from build123d import *

# Parameters (mm, degrees)
SKETCH1_W           = 20
SKETCH1_H           = 20
BOSS_EXTRUDE1_DEPTH = 17
CUT_EXTRUDE1_DEPTH  = 17
SKETCH3_W           = 17
SKETCH3_H           = 13
CUT_EXTRUDE2_DEPTH  = 17
CUT_EXTRUDE3_REACH  = 35
SKETCH4_R           = 3.1
CUT_EXTRUDE4_REACH  = 35
SKETCH5_R           = 3.1


with BuildPart() as part:
    # Sketch1 → Boss-Extrude1 (new body)
    with BuildSketch(Plane(origin=(0, 0, 0), x_dir=(1, 0, 0), z_dir=(0, 1, 0))):
        with Locations((10, 10)):
            Rectangle(SKETCH1_W, SKETCH1_H)
    extrude(amount=BOSS_EXTRUDE1_DEPTH)

    # Sketch2 → Cut-Extrude1 (cut)
    with BuildSketch(Plane(origin=(0, 17, 0), x_dir=(1, 0, 0), z_dir=(0, 1, 0))):
        Polygon((3, 20), (20, 3), (20, 20), align=None)
    extrude(amount=-CUT_EXTRUDE1_DEPTH, mode=Mode.SUBTRACT)

    # Sketch3 → Cut-Extrude2 (cut)
    with BuildSketch(Plane(origin=(0, 0, -20), x_dir=(-1, 0, 0), z_dir=(0, 0, -1))):
        with Locations((-11.5, 8.5)):
            Rectangle(SKETCH3_W, SKETCH3_H)
    extrude(amount=-CUT_EXTRUDE2_DEPTH, mode=Mode.SUBTRACT)

    # Sketch4 → Cut-Extrude3 (cut, up to next)
    with BuildSketch(Plane.ZY, mode=Mode.PRIVATE) as cut_extrude3_sk1:
        with Locations((-10, 8.5)):
            Circle(SKETCH4_R)
    cut_extrude3_tool1 = extrude(cut_extrude3_sk1.sketch, amount=-CUT_EXTRUDE3_REACH, mode=Mode.PRIVATE) & part.part
    add(cut_extrude3_tool1.solids().sort_by_distance((0, 8.5, -10))[0], mode=Mode.SUBTRACT)

    # Sketch5 → Cut-Extrude4 (cut, up to next)
    with BuildSketch(Plane.XY, mode=Mode.PRIVATE) as cut_extrude4_sk1:
        with Locations((10, 8.5)):
            Circle(SKETCH5_R)
    cut_extrude4_tool1 = extrude(cut_extrude4_sk1.sketch, amount=-CUT_EXTRUDE4_REACH, mode=Mode.PRIVATE) & part.part
    add(cut_extrude4_tool1.solids().sort_by_distance((10, 8.5, 0))[0], mode=Mode.SUBTRACT)


solid = part.part
Build history of the part. All positions in model axes, mm. A direction names the side the tool comes from. Round coordinates to 2 decimals unless told otherwise and drop trailing zeros. Order: outer loops, then holes, each group sorted by start corner. A loop starts at its lowest first (then second) coordinate and runs counter-clockwise, first axis right, second up. Notation, with made-up numbers: M 61,51.25 L 108,51.25 A29 ccw 108,77.25 Z; hole C 56,25 d10. An arc over 180 degrees is marked long. Use CSV: the item, a comma, the result in double quotes. Start each with the question number.
(1) Cut at D-D on z = -1.5. List the corners of the cut face in (x, y), then the cut area to 3 significant figures.
(2) Cut at A-A on z = -10. List the corners of the cut face in (x, y), then the cut area to 3 significant figures.
(3) Cut at C-C on y = 8.5. List the corners of the cut face in (x, z), then the cut area to 3 significant figures.
(4) Drill centre lines: probe 1 along Y at (x, z) = (17.75, -4); probe 2 along Y at (x, z) = (1.2, -10); probe 3 along X at (y, z) = (12.5, -9). Where is each one in solid material? Low to high.
(5) Cut at B-B on x = 10. List the corners of the cut face in (y, z), then the cut area to 3 significant figures.
(6) Flat gauge pins, fed straight in: P1, Ø8, axis at y = 8.5, z = -10, coming from the +X side; P2, Ø1, axis at x = 12, y = 12, coming from the -Z side; P3, Ø1.5, axis at x = 9, z = -17, coming from the -Y side. Where does each tip first touch, or does it go through?
(7) Tool access for faces 4 (the face through (20, 8, -1)), 5 (the face through (3, 8, -14)): list every direction of +Z, -Z, +X, -X, +Y, -Y with a clear straight run to the whole face (end or side of a thin tool).
(8) Mould opens along X. For faces 1 (the face through (1.5, 8.6, -13.1)), 2 (the face through (6.9, 8.6, -1.5)), 3 (the face through (11, 16, -12)) say: +X half, -X half, draft (parallel to the pull), parting line (faces both ways), or undercut.
Findings:
1,outline,"M 0,0 L 20,0 L 20,17 L 0,17 Z; hole C 10,8.5 d6.2"
1,area,"310 mm^2"
2,outline,"M 0,0 L 13,0 L 13,2 L 3,2 L 3,5.4 L 0,5.4 Z; M 0,11.6 L 3,11.6 L 3,15 L 13,15 L 13,17 L 0,17 Z"
2,area,"72.4 mm^2"
3,outline,"M 0,-20 L 3,-20 L 3,-13.1 L 0,-13.1 Z; M 0,-6.9 L 3,-6.9 L 3,-3 L 6.9,-3 L 6.9,0 L 0,0 Z; M 13.1,-3 L 20,-3 L 20,0 L 13.1,0 Z"
3,area,"73.8 mm^2"
4,probe 1,"y = 0 to 2, 15 to 17"
4,probe 2,"y = 0 to 5.4, 11.6 to 17"
4,probe 3,"x = 0 to 3"
5,outline,"M 0,-13 L 2,-13 L 2,-3 L 5.4,-3 L 5.4,0 L 0,0 Z; M 11.6,-3 L 15,-3 L 15,-13 L 17,-13 L 17,0 L 11.6,0 Z"
5,area,"72.4 mm^2"
6,P1,"stops at x = 3"
6,P2,"stops at z = -3"
6,P3,"passes through"
7,face 4,"+Z, -Z, +X, +Y, -Y"
7,face 5,"-Z, +X"
8,face 1,"draft"
8,face 2,"undercut"
8,face 3,"+X half"
